Build history of the part. All positions in model axes, mm. A direction names the side the tool comes from. Round coordinates to 2 decimals unless told otherwise and drop trailing zeros. Write each loop counter-clockwise with the first axis right and the second up, starting at its lowest first coordinate (ties: lowest second). Pieces come first, ordered by that corner, then holes.
Item 1: 3-axis set-ups, long thin cutter, end or side, ignore diameter. For faces 5 (the flat face through (15, -1.165, -7)), 6 (the flat face through (18.5, 0, -7)), 7 (the flat face through (-11.5, 0, -7)), 8 (the flat face through (0, 1.167, 2)), 9 (the flat face through (15, 1.165, -7)): which of +Z, -Z, +X, -X, +Y, -Y reach the whole face in a straight line?
Item 2: Drop flat-ended pins along their axis: pin 1 Ø5 at (x, y) = (-5.5, 1.5) entering from +Z; pin 2 Ø7.5 at (x, z) = (-15, -7.5) entering from -Y; pin 3 Ø0.7 at (y, z) = (0.5, 1) entering from -X; pin 4 Ø2 at (x, z) = (16, -8.5) entering from +Y (3 decimals). Give the stop position or say it passes through.
Item 3: Band-saw the part on C-C, the plane z = -5.5. Write the cut outline in (x, y) (3 decimals), then the cut area to 3 significant figures.
Item 4: Wall check: probe 1 along X at (y, z) = (0.1, -8.5); probe 2 along X at (y, z) = (0, 3.5); probe 3 along Z at (x, y) = (-15, 0.55). Give the ranges that are in metal, low to high.
Item 5: Band-saw the part on A-A, the plane y = 0. Write the cut outline in (x, z), then the cut area to 3 significant figures.
Item 6: Band-saw the part on D-D, the plane x = 4. Write the cut outline in (y, z).
Item 7: Mould opens along X. For faces 1 (the cylindrical face through (-15, 0, -12)), 2 (the flat face through (3.5, 0, 2)), 3 (the flat face through (0, 2, 0)), 4 (the flat face through (-3.5, 0, 2)) say: +X half, -X half, draft (parallel to the pull), parting line (faces both ways), or undercut.
Item 8: Band-saw the part on B-B, the plane x = 0. Write the cut outline in (y, z), then the cut area to 3 significant figures.
```python
from build123d import *

# Parameters (mm, degrees)
BOSS_EXTRUDE1_DEPTH = 5
SKETCH3_W           = 7
SKETCH3_H           = 2.333333334
BOSS_EXTRUDE2_DEPTH = 3.5
SKETCH6_W           = 3.5
SKETCH6_H           = 2.333333334
REVOLVE1_ANGLE      = 180
CUT_EXTRUDE1_REACH  = 8.167
SKETCH7_R           = 1
SKETCH8_W           = 7
SKETCH8_H           = 2.33
BOSS_EXTRUDE3_DEPTH = 3.5
SKETCH9_W           = 3.5
SKETCH9_H           = 2.33
REVOLVE2_ANGLE      = 180
SKETCH9_3_W         = 3.5
SKETCH9_3_H         = 2.33
REVOLVE3_ANGLE      = 180
CUT_EXTRUDE2_REACH  = 8.165
SKETCH11_R          = 1


with BuildPart() as part:
    # Sketch2 → Boss-Extrude1 (new body)
    with BuildSketch(Plane.XY):
        with BuildLine():
            Line((-15, -5), (15, -5))
            ThreePointArc((15, -5), (20, 0), (15, 5))
            Line((15, 5), (-15, 5))
            ThreePointArc((-15, 5), (-20, 0), (-15, -5))
        make_face()
    extrude(amount=-BOSS_EXTRUDE1_DEPTH)

    # Sketch3 → Boss-Extrude2 (add)
    with BuildSketch(Plane.XY):
        Rectangle(SKETCH3_W, SKETCH3_H)
    extrude(amount=BOSS_EXTRUDE2_DEPTH)

    # Sketch6 → Revolve1 (revolve)
    with BuildSketch(Plane.XY.offset(3.5)):
        with Locations((-1.75, 0)):
            Rectangle(SKETCH6_W, SKETCH6_H)
    revolve(axis=Axis((0, 1.166666667, 3.5), (0, 1, 0)), revolution_arc=REVOLVE1_ANGLE)

    # Sketch7 → Cut-Extrude1 (cut, up to next)
    with BuildSketch(Plane(origin=(0, 1.166666667, 0), x_dir=(1, 0, 0), z_dir=(0, 1, 0)), mode=Mode.PRIVATE) as cut_extrude1_sk1:
        with Locations((0, -3.5)):
            Circle(SKETCH7_R)
    cut_extrude1_tool1 = extrude(cut_extrude1_sk1.sketch, amount=-CUT_EXTRUDE1_REACH, mode=Mode.PRIVATE) & part.part
    add(cut_extrude1_tool1.solids().sort_by_distance((0, 1.166667, 3.5))[0], mode=Mode.SUBTRACT)

    # Sketch8 → Boss-Extrude3 (add)
    with BuildSketch(Plane(origin=(0, 0, -5), x_dir=(-1, 0, 0), z_dir=(0, 0, -1))):
        with Locations((-15, 0)):
            Rectangle(SKETCH8_W, SKETCH8_H)
        with Locations((15, 0)):
            Rectangle(SKETCH8_W, SKETCH8_H)
    extrude(amount=BOSS_EXTRUDE3_DEPTH)

    # Sketch9 → Revolve2 (revolve)
    with BuildSketch(Plane(origin=(0, 0, -8.5), x_dir=(-1, 0, 0), z_dir=(0, 0, -1))):
        with Locations((-16.75, 0)):
            Rectangle(SKETCH9_W, SKETCH9_H)
    revolve(axis=Axis((15, 1.165, -8.5), (0, 1, 0)), revolution_arc=REVOLVE2_ANGLE)

    # Sketch9_3 → Revolve3 (revolve)
    with BuildSketch(Plane(origin=(0, 0, -8.5), x_dir=(-1, 0, 0), z_dir=(0, 0, -1))):
        with Locations((13.25, 0)):
            Rectangle(SKETCH9_3_W, SKETCH9_3_H)
    revolve(axis=Axis((-15, 1.165, -8.5), (0, 1, 0)), revolution_arc=REVOLVE3_ANGLE)

    # Sketch11 → Cut-Extrude2 (cut, up to next)
    with BuildSketch(Plane(origin=(0, 1.165, 0), x_dir=(1, 0, 0), z_dir=(0, 1, 0)), mode=Mode.PRIVATE) as cut_extrude2_sk1:
        with Locations((-15, 8.5)):
            Circle(SKETCH11_R)
    cut_extrude2_tool1 = extrude(cut_extrude2_sk1.sketch, amount=-CUT_EXTRUDE2_REACH, mode=Mode.PRIVATE) & part.part
    add(cut_extrude2_tool1.solids().sort_by_distance((-15, 1.165, -8.5))[0], mode=Mode.SUBTRACT)
    # Sketch11 → Cut-Extrude2 (cut, up to next)
    with BuildSketch(Plane(origin=(0, 1.165, 0), x_dir=(1, 0, 0), z_dir=(0, 1, 0)), mode=Mode.PRIVATE) as cut_extrude2_sk2:
        with Locations((15, 8.5)):
            Circle(SKETCH11_R)
    cut_extrude2_tool2 = extrude(cut_extrude2_sk2.sketch, amount=-CUT_EXTRUDE2_REACH, mode=Mode.PRIVATE) & part.part
    add(cut_extrude2_tool2.solids().sort_by_distance((15, 1.165, -8.5))[0], mode=Mode.SUBTRACT)


solid = part.part
```
Results:
1. face 5: -Z, +X, -X, -Y
1. face 6: -Z, +X, +Y, -Y
1. face 7: -Z, +Y, -Y
1. face 8: +Z, +X, -X, +Y
1. face 9: -Z, +X, -X, +Y
2. pin 1: stops at z = 5.27
2. pin 2: stops at y = -5
2. pin 3: stops at x = -3.5
2. pin 4: stops at y = 1.165
3. outline: (-18.5, -1.165) - (-11.5, -1.165) - (-11.5, 1.165) - (-18.5, 1.165) - close; (11.5, -1.165) - (18.5, -1.165) - (18.5, 1.165) - (11.5, 1.165) - close
3. area: 32.6 mm2
4. probe 1: x = -18.5 to -16, -14 to -11.5, 11.5 to 14, 16 to 18.5
4. probe 2: x = -3.5 to -1, 1 to 3.5
4. probe 3: z = -12 to -9.5, -7.5 to 0
5. outline: (-20, -5) - (-18.5, -5) - (-18.5, -8.5) arc R3.5 ccw to (-11.5, -8.5) - (-11.5, -5) - (11.5, -5) - (11.5, -8.5) arc R3.5 ccw to (18.5, -8.5) - (18.5, -5) - (20, -5) - (20, 0) - (3.5, 0) - (3.5, 3.5) arc R3.5 ccw to (-3.5, 3.5) - (-3.5, 0) - (-20, 0) - close; hole circle Ø2 at (-15, -8.5); hole circle Ø2 at (0, 3.5); hole circle Ø2 at (15, -8.5)
5. area: 322 mm2
6. outline: (-5, -5) - (5, -5) - (5, 0) - (-5, 0) - close
7. face 1: undercut
7. face 2: +X half
7. face 3: draft
7. face 4: -X half
8. outline: (-5, -5) - (5, -5) - (5, 0) - (1.17, 0) - (1.17, 2.5) - (-1.17, 2.5) - (-1.17, 0) - (-5, 0) - close; (-1.17, 4.5) - (1.17, 4.5) - (1.17, 7) - (-1.17, 7) - close
8. area: 61.7 mm2
